Autodesk Inventor part; units mm, degrees
ref_plane "YZ Plane" through (0, 0, 0) normal (1, 0, 0) x (0, 1, 0)
ref_plane "XZ Plane" through (0, 0, 0) normal (0, 1, 0) x (-1, 0, 0)
ref_plane "XY Plane" through (0, 0, 0) normal (0, 0, 1) x (1, 0, 0)
sketch "Sketch2" plane through (0, 0, 0) normal (1, 0, 0) x (0, 1, 0)
  line L0 (127.2876, 96.9132) -> (-12.7124, 96.9132) construction
  line L1 (-12.7124, 96.9132) -> (-12.7124, -363.0868) construction
  line L2 (-12.7124, -363.0868) -> (127.2876, -363.0868) construction
  line L3 (127.2876, -363.0868) -> (127.2876, 96.9132) construction
  line L4 (97.2876, 66.9132) -> (17.2876, 66.9132) construction
  line L5 (17.2876, 66.9132) -> (17.2876, -333.0868) construction
  line L6 (17.2876, -333.0868) -> (97.2876, -333.0868) construction
  line L7 (97.2876, -333.0868) -> (97.2876, 66.9132) construction
  point P0 (0, 0)
  dimension "d2" = 140
  dimension "d3" = 460
  dimension "d4" = 80
  dimension "d5" = 400
  dimension "d6" = 30
  dimension "d7" = 30
sketch "Sketch3" plane through (0, 0, 0) normal (1, 0, 0) x (0, 1, 0)
  circle A0 centre (-62.7124, 66.9132) radius 20
  line L0 (-12.7124, 96.9132) -> (-12.7124, -363.0868) construction
  circle A1 centre (-62.7124, -13.0868) radius 20
  circle A2 centre (-62.7124, -93.0868) radius 20
  circle A3 centre (-62.7124, -173.0868) radius 20
  circle A4 centre (-62.7124, -253.0868) radius 20
  circle A5 centre (-62.7124, -333.0868) radius 20
  line L1 (127.2876, 96.9132) -> (-12.7124, 96.9132) construction
  point P0 (0, 0)
  dimension "d8" = 40
  dimension "d9" = 50
  dimension "d12" = 80
  dimension "d17" = 30
sketch "Sketch1" plane through (0, 0, 0) normal (1, 0, 0) x (0, 1, 0)
  circle A0 centre (45.5719, 146.9132) radius 40
  circle A1 centre (85.5719, -453.0868) radius 40
  line L0 (127.2876, 96.9132) -> (-12.7124, 96.9132) construction
  line L1 (-12.7124, -363.0868) -> (127.2876, -363.0868) construction
  line L2 (-62.7124, 66.9132) -> (-62.7124, -13.0868) construction
  line L3 (-62.7124, -253.0868) -> (-62.7124, -333.0868) construction
  line L4 (85.2399, 141.7706) -> (125.4799, -450.3748) construction
  circle A2 centre (-62.7124, 66.9132) radius 20
  line L5 (17.2876, 175.1975) -> (-76.8545, 81.0553)
  circle A3 centre (-62.7124, -333.0868) radius 20
  line L6 (-76.8545, -347.2289) -> (57.2876, -481.3711) construction
  point P0 (0, 0)
  dimension "d0" = 80
  dimension "d1" = 80
  dimension "d18" = 50
  dimension "d19" = 90
  dimension "d45" = 135
  dimension "d46" = 135
sketch "Sketch4" plane through (0, 0, 0) normal (1, 0, 0) x (0, 1, 0)
  line L0 (37.6815, -3.0868) -> (-57.7124, 26.9132) construction
  circle A0 centre (-62.7124, 66.9132) radius 20
  circle A1 centre (-62.7124, -13.0868) radius 20
  line L1 (-62.7124, 66.9132) -> (-62.7124, -13.0868) construction
  circle A2 centre (-27.7124, 112.5679) radius 20 construction
  circle A3 centre (-27.7124, 32.5679) radius 20 construction
  line L2 (-27.7124, 72.5679) -> (37.6815, -3.0868) construction
  line L3 (-27.7124, 72.5679) -> (-57.7124, 26.9132) construction
  line L4 (37.6815, -3.0868) -> (-42.7124, 49.7406) construction
  line L5 (-12.7124, 96.9132) -> (-12.7124, -363.0868) construction
  point P0 (0, 0)
  point P1 (-61.7124, 47.9132)
  point P2 (83.0715, 79.9132)
  point P3 (83.0715, -80.0868)
  point P4 (37.6815, -163.0868)
  point P5 (83.0715, -240.0868)
  point P6 (37.6815, -323.0868)
  dimension "d22" = 40
  dimension "d23" = 5
  dimension "d24" = 30
  dimension "d25" = 40
  dimension "d26" = 40
  dimension "d27" = 80
  dimension "d28" = 40
  dimension "d29" = 100
  dimension "d30" = 100
  dimension "d31" = 35
  dimension "d32" = 54.6292
  dimension "d33" = 27.3146
  dimension "d34" = 56.691
  dimension "d35" = 95.3939
  dimension "d36" = 45.39
  dimension "d37" = 83
  dimension "d40" = 160
sketch "Sketch6" plane through (0, 0, 0) normal (1, 0, 0) x (0, 1, 0)
  line L0 (234.6261, -208.0868) -> (-157.479, -208.0868) construction
  line L1 (237.7494, -58.0868) -> (-154.3557, -58.0868) construction
  line L2 (17.2876, -333.0868) -> (97.2876, -333.0868) construction
  line L3 (97.2876, 66.9132) -> (17.2876, 66.9132) construction
  point P0 (0, 0)
  dimension "d61" = 125
  dimension "d62" = 125
sketch "Sketch5" plane through (0, 0, 0) normal (1, 0, 0) x (0, 1, 0)
  arc A0 (90.5716, 146.9132) -> (47.894, 164.5909) centre (65.5716, 146.9132) ccw
  arc A1 (47.894, 164.5909) -> (90.5716, 146.9132) centre (65.5716, 146.9132) ccw construction
  line L0 (114.7874, 96.9132) -> (-25.2126, 96.9132) construction
  line L1 (-32.7126, -363.0868) -> (107.2874, -363.0868) construction
  line L2 (217.7491, -58.0868) -> (-174.356, -58.0868) construction
  line L3 (214.6258, -208.0868) -> (-177.4793, -208.0868) construction
  circle A2 centre (65.5716, 146.9132) radius 11
  circle A3 centre (65.5716, 146.9132) radius 55 construction
  line L4 (-9.4284, 107.2685) -> (47.894, 164.5909)
  line L5 (-2.7126, 66.9132) -> (-2.7126, -333.0868) construction
  line L6 (-62.7124, -13.0868) -> (-62.7124, -93.0868) construction
  line L7 (-62.7124, -173.0868) -> (-62.7124, -253.0868) construction
  line L8 (90.5716, -363.0868) -> (90.5716, 146.9132)
  line L9 (90.5716, -363.0868) -> (90.5716, -366.2493)
  arc A4 (82.3188, -373.7114) -> (90.5716, -366.2493) centre (83.0716, -366.2493) ccw
  arc A5 (12.4757, -366.2343) -> (14.9188, -366.9114) centre (15.6716, -359.4493) ccw
  line L10 (82.3188, -373.7114) -> (14.9188, -366.9114)
  arc A6 (-7.9036, -348.1319) -> (-0.1706, -360.2774) centre (5.5716, -348.0868) ccw
  line L11 (12.4757, -366.2343) -> (-0.1706, -360.2774)
  line L12 (-7.9036, -348.1319) -> (-9.4284, 107.2685)
  point P0 (0, 0)
  point P1 (83.0716, 81.9132)
  point P2 (83.0716, -348.0868)
  point P3 (16.3276, 122.4179)
  point P4 (8.0719, -82.4742)
  point P5 (8.0719, -243.0868)
  point P6 (-17.7126, -58.0868)
  point P7 (-17.7126, -208.0868)
  point P8 (5.5716, 81.9132)
  point P9 (-62.7124, 66.9132)
  point P10 (-62.7124, -333.0868)
  point P11 (-62.7124, -53.0868)
  point P12 (-62.7124, -213.0868)
  point P13 (2.2876, 6.9132)
  point P14 (42.2876, 26.9132)
  point P15 (47.2876, -93.0868)
  point P16 (7.2876, -113.0868)
  point P17 (7.2876, -153.0868)
  point P18 (47.2876, -173.0868)
  point P19 (42.2876, -293.0868)
  point P20 (2.2876, -273.0868)
  point P21 (2.2876, 6.9132)
  point P22 (-62.7124, 66.9132)
  point P23 (5.5716, -208.0868)
  point P24 (5.5716, -58.0868)
  point P25 (73.0216, -4.2568)
  point P26 (78.0216, -124.2568)
  point P27 (78.0216, -141.9168)
  point P28 (73.0216, -261.9168)
  dimension "d84" = 110
  dimension "d47" = 50
  dimension "d63" = 15
  dimension "d65" = 15
  dimension "d81" = 22
  dimension "d101" = 7.5
  dimension "d151" = 15
  dimension "d155" = 15
  dimension "d159" = 15
  dimension "d163" = 60
  dimension "d164" = 65
  dimension "d165" = 20
  dimension "d166" = 40
  dimension "d174" = 60
  dimension "d175" = 70
  dimension "d176" = 40
  dimension "d177" = 20
  dimension "d196" = 128.284
  dimension "d198" = 11.17
  dimension "d199" = 70.734
  dimension "d200" = 11.17
  dimension "d201" = 70.734
  dimension "d204" = 11.17
  dimension "d213" = 65
  dimension "d214" = 40
  dimension "d215" = 20
  dimension "d216" = 20
  dimension "d217" = 40
  dimension "d218" = 70.734
  dimension "d219" = 70.734
  dimension "d220" = 11.17
  dimension "d221" = 67.4
  dimension "d222" = 6.8
  dimension "d223" = 7.5
  dimension "d224" = 15
  dimension "d225" = 15
extrude "Extrusion1" add sketch "Sketch5" against normal blind 5
hole "Hole1" at (0, 83.0716, 81.9132) at (0, 16.3276, 122.4179) at (0, 5.5716, -348.0868) at (0, 83.0716, -348.0868) at (0, -17.7126, -58.0868) at (0, -17.7126, -208.0868) at (0, 5.5716, 81.9132) at (0, 5.5716, -58.0868) at (0, 5.5716, -208.0868) direction (-1, 0, 0) diameter 5 end through all
hole "Otwór2" at (0, 2.2876, 6.9132) at (0, 42.2876, 26.9132) at (0, 7.2876, -113.0868) at (0, 47.2876, -93.0868) at (0, 7.2876, -153.0868) at (0, 47.2876, -173.0868) at (0, 2.2876, -273.0868) at (0, 42.2876, -293.0868) at (0, 83.0716, -366.2493) direction (-1, 0, 0) diameter 6 end through all
hole "Otwór3" at (0, 73.0216, -4.2568) at (0, 78.0216, -141.9168) at (0, 78.0216, -124.2568) at (0, 73.0216, -261.9168) at (0, 15.6716, -359.4493) direction (-1, 0, 0) diameter 5 end through all
equation "\"d28\" = 0.5 * d27"
equation "\"d30\" = d29"
equation "\"d33\" = 0.5 * d32"
equation "\"d62\" = d61"
properties part number "plyta_glowna" material "Aluminium 6061"
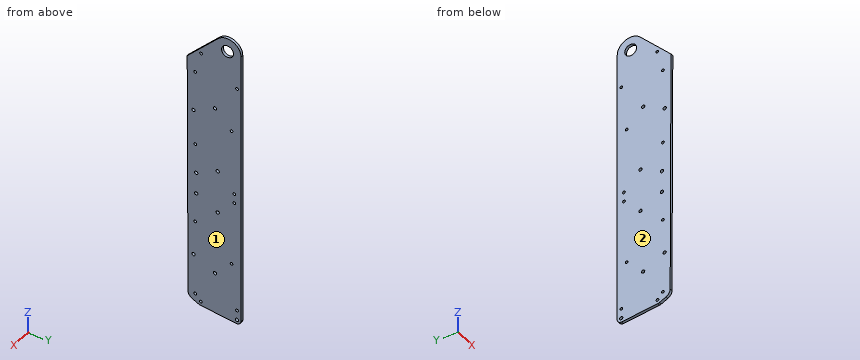
Input: part model. Units: mm. Frame: model coordinates. Face numbers are marked on the shaded views. Give positions to 0.01 mm unless a question says otherwise; leave off trailing zeros. Order: outer loops, then holes, each group sorted by start corner. A loop starts at its lowest first (then second) coordinate and runs counter-clockwise, first axis right, second up. Notation, with made-up numbers: (19.25, 41) - (65.25, 41) arc R15 cw to (65.25, 66) - close; hole circle Ø1 at (79, -9). An arc over 180 degrees is marked (long way). Put each result on its own line as item: value.
Item 1: Draft query along X for the marked faces 1 and 2. Return one class per face: +X half, -X half, draft (parallel to the pull), parting line (faces both ways), or undercut.
Found:
face 1: +X half
face 2: -X half
Item 2: Section query A-A, the plane x = -3.9. Count the separate pieces of the cut face and the enclosed holes in it, then the cut area to 3 significant figures.
Found:
separate pieces: 1
enclosed holes: 22
area: 50,500 mm^2
Item 3: Ray query, L1, parallel to Z at x = -3.25, y = 43.5; L2, parallel to Z at x = -1.15, y = 2; L3, parallel to Z at x = -4.45, y = 82. Return the intervals inside material, ascending. Write a range as from..to.
Found:
L1: z = -369.79..-295.83, -290.34..24.17, 29.66..160.2
L2: z = -361.3..-276.07, -270.1..3.93, 9.9..118.7
L3: z = -373.68..-369.05, -363.45..-350.35, -345.83..79.65, 84.17..165.76
Item 4: Section query B-B, the plane y = 24. Return loops of the section in (x, z).
Found:
outline: (-5, -367.83) - (0, -367.83) - (0, 140.7) - (-5, 140.7) - close
Item 5: Contact query for flat-ended pins moving along their axis: pin 1 (4 mm diameter, centred on y = 16.33, z = 122.42, fed in from +X); pin 2 (1.5 mm diameter, centred on x = -3.5, y = 5.5, fed in from -Z). Output: stop coordinate, or through.
Found:
pin 1: passes through
pin 2: stops at z = -363.3
